Input: part model. Units: mm. Frame: model coordinates. A direction names the side the tool comes from. Coordinates: 2 decimals unless noted, no trailing zeros. Write each loop counter-clockwise with the first axis right and the second up, starting at its lowest first coordinate (ties: lowest second). Pieces come first, ordered by that corner, then holes. Notation, with made-up numbers: (41, 14) - (78, 14) arc R20 ccw to (78, 35) - close; hole circle Ø7 at (27.5, 36.5). An arc over 180 degrees is marked (long way). Use a Markdown table: item, result. Add a question column.
Q1. Material intervals for probe 1 along Y at (x, z) = (63, 9.6); probe 2 along Y at (x, z) = (65, 14); probe 3 along Z at (x, y) = (6, 51), sorted ascending. Write a range as from..to.
Q2. Set-up query: faces 4 (the face through (83.944, 13.648, 8.974)), 5 (the face through (4.056, 16.352, 8.974)), 6 (the face through (46, 55, 3)), 7 (the face through (29, 5, 4)). Return all of +Z, -Z, +X, -X, +Y, -Y with unobstructed straight access to the full face (end or side cutting, diameter ignored); none if empty.
Q3. Mould query, pull axis Y, two halves, no side actions, for faces 1 (the face through (43, 60, 4)), 2 (the face through (54.224, 28.639, 11.042)), 3 (the face through (45, 24, 15)). Classes: released by +Y, released by -Y, zero draft, split by the parting line, or undercut.
Q4. Pin query (flat end, axial travel): P1, Ø6.5, axis at x = 7, y = 55, coming from the -Z side; P2, Ø1, axis at x = 26.5, z = 13.5, coming from the -Y side; P3, Ø4, axis at x = 39.5, z = 12, coming from the +Y side; P4, Ø6.5, axis at x = 27, y = 5, coming from the +Z side. Return the tip coordinate at first contact, or that it passes through.
Q5. Section query A-A (z = 11). Return the cut outline in (x, y), then the cut area to 3 significant figures.
Q6. Section query B-B (z = 3.5). Give the number of separate pieces and of enclosed holes in the cut face, then the cut area to 3 significant figures.
Autodesk Inventor part; units mm, degrees
ref_plane "Work Plane1" through (44, 60, 0) normal (1, 0, 0) x (0, 0, -1)
ref_plane "YZ Plane" through (0, 0, 0) normal (1, 0, 0) x (0, 1, 0)
ref_plane "XZ Plane" through (0, 0, 0) normal (0, 1, 0) x (-1, 0, 0)
sketch "Sketch1" plane through (0, 0, 0) normal (0, 0, 1) x (1, 0, 0)
  line L0 (0, 0) -> (88, 0)
  line L1 (88, 0) -> (88, 10)
  line L2 (88, 10) -> (0, 10)
  line L3 (0, 10) -> (0, 0)
  dimension "d0" = 88
  dimension "d1" = 10
extrude "Extrusion1" add sketch "Sketch1" along normal blind 5
sketch "Sketch2" plane through (0, 10, 0) normal (0, 1, 0) x (1, 0, 0)
  line L0 (0, 0) -> (88, 0)
  line L1 (88, 0) -> (88, -15)
  line L2 (88, -15) -> (0, -15)
  line L3 (0, -15) -> (0, 0)
  dimension "d4" = 88
  dimension "d5" = 15
extrude "Extrusion2" add sketch "Sketch2" along normal blind 50
sketch "Sketch4" plane through (0, 0, 0) normal (0, 0, -1) x (-1, 0, 0)
  line L0 (0, 0) -> (-88, 0)
  line L1 (-88, 0) -> (-88, 10)
  line L2 (-88, 10) -> (0, 10)
  line L3 (0, 10) -> (0, 0)
  point P0 (-78, 5)
  dimension "d10" = 10
  dimension "d11" = 5
hole "Hole1" at (78, 5, 0) direction (0, 0, 1) diameter 4 depth 10 tip angle 120 countersink diameter 8 countersink angle 90
pattern_linear "Rectangular Pattern1" count 5 spacing 17 along (-1, 0, 0) of "Hole1"
sketch "Sketch5" plane through (88, 0, 5) normal (1, 0, 0) x (0, 0, -1)
  line L0 (0, 10) -> (-10, 10)
  line L1 (-10, 10) -> (-10, 60)
  point P0 (5, 0)
  point P1 (-2.5, 15)
  dimension "d22" = 5
  dimension "d23" = 7.5
hole "Hole2" at (88, 15, 7.5) direction (-1, 0, 0) diameter 4 depth 8 tip angle 120
thread "Thread1"
pattern_linear "Rectangular Pattern2" count 3 spacing 18 along (0, 1, 0) of "Hole2"
ref_plane "Work Plane1" through (44, 60, 0) normal (1, 0, 0) x (0, 0, -1)
mirror "Mirror1" about plane through (44, 60, 0) normal (1, 0, 0) of "Hole2", "Rectangular Pattern2"
sketch "Sketch6" plane through (0, 10, 15) normal (0, 0, 1) x (1, 0, 0)
  circle A0 centre (25, 15) radius 9.5
  line L0 (0, 50) -> (88, 50)
  line L1 (0, -10) -> (88, -10)
  point P0 (44, 50)
  dimension "d36" = 19
  dimension "d47" = 19
  dimension "d48" = 25
extrude "Extrusion3" cut sketch "Sketch6" against normal blind 7
sketch "Sketch7" plane through (25, 25, 8) normal (0, 0, 1) x (1, 0, 0)
  circle A0 centre (0, 0) radius 9.5
  circle A1 centre (0, 0) radius 3.5
  point P0 (-25, -25)
  dimension "d39" = 7
extrude "Extrusion4" cut sketch "Sketch7" against normal blind 58.5 and the other way blind 29.25 contours A1
chamfer "Chamfer1" distance 1 angle 45 1 edges at (15.5, 25, 15)
mirror "Mirror2" about plane through (44, 60, 0) normal (1, 0, 0) of "Extrusion4", "Extrusion3", "Chamfer1"
sketch "Sketch8" plane through (0, 60, 0) normal (0, 1, 0) x (1, 0, 0)
  line L0 (88, 0) -> (0, 0)
  line L1 (0, 0) -> (0, -15)
  line L2 (0, -15) -> (88, -15)
  line L3 (88, -15) -> (88, 0)
  line L4 (0, -15) -> (88, -15)
  line L5 (88, -15) -> (88, -7.5)
  line L6 (88, -7.5) -> (0, -7.5)
  line L7 (0, -7.5) -> (0, -15)
extrude "Extrusion5" cut sketch "Sketch8" against normal blind 3 contours L3 L2 L1 L6
sketch "Sketch9" plane through (0, 0, 0) normal (0, 0, -1) x (-1, 0, 0)
  circle A0 centre (-81, 55) radius 2
  circle A1 centre (-44, 55) radius 2
  circle A2 centre (-7, 55) radius 2
  point P0 (0, 0)
hole "Hole3" at (81, 55, 0) at (44, 55, 0) at (7, 55, 0) direction (0, 0, 1) diameter 4 depth 6.5 tip angle 120
sketch "Sketch10" plane through (88, 0, 5) normal (1, 0, 0) x (0, 0, -1)
  line L0 (-2.5, 60) -> (-2.5, 57)
  line L1 (-2.5, 57) -> (-10, 57)
  line L2 (-10, 10) -> (-10, 57)
  line L3 (0, 10) -> (-10, 10)
  line L4 (0, 0) -> (0, 10)
  line L5 (5, 0) -> (0, 0)
  line L6 (5, 0) -> (5, 60)
  line L7 (-2.5, 60) -> (5, 60)
  circle A0 centre (-2.5, 15) radius 2
  circle A1 centre (-2.5, 33) radius 2
  circle A2 centre (-2.5, 51) radius 2
  line L8 (-10, 41) -> (-3, 41)
  line L9 (-3, 41) -> (-3, 38)
  line L10 (-3, 38) -> (-10, 38)
  line L11 (-10, 38) -> (-10, 41)
  dimension "d58" = 7
  dimension "d59" = 3
  dimension "d60" = 28
extrude "Extrusion6" cut sketch "Sketch10" against normal blind 114.5 contours L8 L9 L10 L2
equation "\"d21\" = hole_step"
equation "\"hole_l_offset\" = 10"
equation "\"hole_step\" = 17"
equation "\"hole_h_offset\" = 5"
properties part number "КВ33.000.102 - Стенка толстая" material "Steel"
Values follow:
| question | item | result |
|---|---|---|
| 1 | probe 1 | 10..15.5, 34.5..38, 41..57 |
| 1 | probe 2 | 10..15.71, 34.29..38, 41..57 |
| 1 | probe 3 | 0..5.5, 9.5..15 |
| 2 | face 4 | +X |
| 2 | face 5 | -X |
| 2 | face 6 | -Z |
| 2 | face 7 | +Z, -Z |
| 3 | face 1 | released by +Y |
| 3 | face 2 | undercut |
| 3 | face 3 | zero draft |
| 4 | P1 | z = 0 |
| 4 | P2 | y = 10 |
| 4 | P3 | y = 57 |
| 4 | P4 | z = 5 |
| 5 | outline | (0, 10) - (88, 10) - (88, 38) - (0, 38) - close; (0, 41) - (88, 41) - (88, 57) - (0, 57) - close; hole circle Ø19 at (25, 25); hole circle Ø19 at (63, 25) |
| 5 | area | 3,300 mm2 |
| 6 | separate pieces | 1 |
| 6 | enclosed holes | 10 |
| 6 | area | 5,100 mm2 |
